from build123d import *

# Parameters (mm, degrees)
F0_W     = 80
F0_H     = 13
F2_W     = 80
F2_H     = 18
F4_T     = -1.5
F5_W     = 68
F5_H     = 34.3112887415
F6_DEPTH = 2.7
F7_W     = 44
F7_H     = 11.5
F8_DEPTH = 25
F9_R     = 0.74999


# Not quite as in the source:
# - a fillet or chamfer is up to 0.001 mm smaller than in the source, because OpenCascade refuses the exact size


with BuildPart() as f3:
    # F0 (on Top) → F3 section 0
    with BuildSketch(Plane.XY):
        with Locations((40, -6.5)):
            Rectangle(F0_W, F0_H)
    # F2 (on offset) → F3 section 1
    with BuildSketch(Plane.XY.offset(40)):
        with Locations((40, -9)):
            Rectangle(F2_W, F2_H)
    loft()

    # F4
    f4_openings = [f3.faces().sort_by_distance(p)[0] for p in [
        (40, -9, 40),
    ]]
    offset(amount=F4_T, openings=f4_openings)

    # F5 (on face) → F6 (cut)
    with BuildSketch(Plane(origin=(0, -12.8, -1.6), x_dir=(1, 0, 0), z_dir=(0, -0.9922778767, -0.1240347346))):
        with Locations((40, 24.7680959204)):
            Rectangle(F5_W, F5_H)
    extrude(amount=-F6_DEPTH, mode=Mode.SUBTRACT)

    # F7 (on face) → F8 (cut)
    with BuildSketch(Plane(origin=(0, 0, 0), x_dir=(1, 0, 0), z_dir=(0, 0, -1))):
        with Locations((40, 7.25)):
            Rectangle(F7_W, F7_H)
    extrude(amount=-F8_DEPTH, mode=Mode.SUBTRACT)

    # F9 (radius 0.75 in the source; OpenCascade refuses exactly that, so slightly less here)
    f9_edges = [f3.edges().sort_by_distance(p)[0] for p in [
        (80, -15.5, 20),
        (80, -6.5, 0),
        (80, 0, 20),
        (0, -15.5, 20),
        (0, 0, 20),
        (0, -6.5, 0),
        (6, -15.872104, 22.976834),
        (74, -15.872104, 22.976834),
        (3, -18, 40),
        (77, -18, 40),
        (80, -9, 40),
        (74, -17.244163, 40),
        (0, -9, 40),
        (40, 0, 40),
        (3.75, -16.488327, 40),
        (1.5, -8.994163, 40),
        (40, -1.5, 40),
        (78.5, -8.994163, 40),
        (76.25, -16.488327, 40),
        (12, -12.255792, 6.139719),
        (68, -12.255792, 6.139719),
    ]]
    fillet(f9_edges, radius=F9_R)


solid = f3.part
Here's how the part is built. I have some questions about the finished solid (model axes, mm). A direction names the side the tool comes from. Coordinates: 2 decimals unless noted, no trailing zeros.
Item 1: I need wall thicknesses on line 1 (X direction, y = -5.25, z = 10); line 2 (Y direction, x = 71, z = 28.5); line 3 (Z direction, x = 75.5, y = -8.5). Which ranges of each line are inside material? Lowest first, please.
Result sheet:
line 1: x = 0 to 1.5, 78.5 to 80
line 2: y = -1.5 to 0
line 3: z = 0 to 1.5
Item 2: If we mould it in two halves opening along X, with no side actions, what happens to faces 1 (the face through (10, -7, 1.5)), 2 (the face through (74.23, -15.64, 22.81)), 3 (the face through (34.002, -13.465, 3.717))? For each: +X half, -X half, draft (parallel to the pull), parting line (faces both ways), or undercut.
Result sheet:
face 1: undercut
face 2: undercut
face 3: draft
Item 3: For faces 4 (the face through (62, -8, 1)), 5 (the face through (41, 0, 20)), 6 (the face through (78.5, -8, 21)), which set-ups out of +Z, -Z, +X, -X, +Y, -Y let a thin tool reach every point of the face, with its end or its side?
Result sheet:
face 4: +Z, -Z
face 5: +Z, -Z, +X, -X, +Y
face 6: +Z
Item 4: For P1, Ø8, axis at x = 58.5, z = 16, coming from the -Y side; P2, Ø12, axis at x = 22.5, z = 10, coming from the -Y side; P3, Ø1, axis at x = 12, y = -4.5, coming from the +Z side, each with a flat end and sliding along its axis, tell me the tip position at first contact or that it passes through.
Result sheet:
P1: stops at y = -1.5
P2: stops at y = -13.74
P3: stops at z = 1.5
